```python
from build123d import *

# Parameters (mm, degrees)
BOSS_EXTRUDE4_DEPTH = 50
SKETCH7_R           = 1.75
CUT_EXTRUDE1_DEPTH  = 17.825


with BuildPart() as part:
    # Sketch6 → Boss-Extrude4 (new body)
    with BuildSketch(Plane.XZ):
        with BuildLine():
            Line((-1, 25.784833184), (-1, 12.785954208))
            ThreePointArc((-1, 12.785954208), (-12.825, 0), (-1, -12.785954208))
            Line((-1, -12.785954208), (-1, -25.784833184))
            Line((-1, -25.784833184), (-6, -25.784833184))
            Line((-6, -25.784833184), (-6, -16.784833184))
            ThreePointArc((-6, -16.784833184), (-17.825, 0), (-6, 16.784833184))
            Line((-6, 16.784833184), (-6, 25.784833184))
            Line((-6, 25.784833184), (-1, 25.784833184))
        make_face()
    extrude(amount=BOSS_EXTRUDE4_DEPTH)

    # Sketch7 → Cut-Extrude1 (cut, through all)
    with BuildSketch(Plane(origin=(-1, 0, 0), x_dir=(0, 0, -1), z_dir=(1, 0, 0))):
        with Locations((-19.285393696, -10)):
            Circle(SKETCH7_R)
        with Locations((-19.285393696, -40)):
            Circle(SKETCH7_R)
        with Locations((19.285393696, -40)):
            Circle(SKETCH7_R)
        with Locations((19.285393696, -10)):
            Circle(SKETCH7_R)
    extrude(amount=-CUT_EXTRUDE1_DEPTH, mode=Mode.SUBTRACT)


solid = part.part
```
Geometry: final body of the model. Coordinates: model frame, mm. A direction names the side the tool comes from. Coordinates: 2 decimals unless noted, no trailing zeros. Order: outer loops, then holes, each group sorted by start corner. A loop starts at its lowest first (then second) coordinate and runs counter-clockwise, first axis right, second up. Notation, with made-up numbers: (87, 33.5) - (95, 33.5) arc R12 ccw to (95, 43.5) - close; hole circle Ø11 at (-12.5, 0). An arc over 180 degrees is marked (long way). Write each question's results on one line, items separated by ' | '.
1) Section B-B, the plane x = -9.5. Return loops of the section in (y, z).
Results list:
outline: (-50, -15.08) - (0, -15.08) - (0, -8.62) - (-50, -8.62) - close; (-50, 8.62) - (0, 8.62) - (0, 15.08) - (-50, 15.08) - close
2) Set-up query: faces 4 (the flat face through (-6, -25, 21)), 5 (the cylindrical face through (-3.465, -9.474, -20.955)), 6 (the flat face through (-6, -25, -21)). Return all of +Z, -Z, +X, -X, +Y, -Y with unobstructed straight access to the full face (end or side cutting, diameter ignored); none if empty.
Results list:
face 4: +Z, -X, +Y, -Y | face 5: +X, -X | face 6: -Z, -X, +Y, -Y
3) Line query: line 1 (X direction, y = -28, z = -18); line 2 (Z direction, x = -9, y = -43); line 3 (Z direction, x = -2.75, y = -23). Output: solid intervals per line, ascending. Write a range as from..to.
Results list:
line 1: -6..-1 | line 2: -15.39..-9.14, 9.14..15.39 | line 3: -25.78..-12.53, 12.53..25.78
4) Pull-direction query (Z, two-part tool) for faces 1 (the flat face through (-3, -25, -25.785)), 2 (the cylindrical face through (-3.5, -41.7, 19.7)), 3 (the flat face through (-1, -25, -19)); classes: pulls with the +Z half, pulls with the -Z half, needs draft (parallel to the pull), parting line crosses it, or undercut.
Results list:
face 1: pulls with the -Z half | face 2: undercut | face 3: needs draft
5) Pin query (flat end, axial travel): pin 1 (4 mm diameter, centred on y = -29, z = 13, fed in from -X); pin 2 (4.5 mm diameter, centred on y = -34.5, z = -22, fed in from -X); pin 3 (2 mm diameter, centred on y = -40, z = -19.29, fed in from +X); pin 4 (2 mm diameter, centred on x = -16, y = -32, fed in from -Z). Return the tip coordinate at first contact, or that it passes through.
Results list:
pin 1: x = -14.03 | pin 2: x = -6 | pin 3: through | pin 4: z = -9.63
6) Section A-A, the plane y = -40. Return loops of the section in (x, z) (3 decimals), plus the area to 3 significant figures.
Results list:
outline: (-6, -25.785) - (-1, -25.785) - (-1, -21.035) - (-6, -21.035) - close; (-6, -17.535) - (-1, -17.535) - (-1, -12.786) arc R12.825 cw to (-1, 12.786) - (-1, 17.535) - (-6, 17.535) - (-6, 16.785) arc R17.825 ccw to (-6, -16.785) - close; (-6, 21.035) - (-1, 21.035) - (-1, 25.785) - (-6, 25.785) - close | area: 279 mm^2
7) Section C-C, the plane x = -4.25. Return loops of the section in (y, z), plus the area to 3 significant figures.
Results list:
outline: (-50, -25.78) - (0, -25.78) - (0, -12.1) - (-50, -12.1) - close; (-50, 12.1) - (0, 12.1) - (0, 25.78) - (-50, 25.78) - close; hole circle Ø3.5 at (-40, -19.29); hole circle Ø3.5 at (-40, 19.29); hole circle Ø3.5 at (-10, -19.29); hole circle Ø3.5 at (-10, 19.29) | area: 1,330 mm^2
8) Section D-D, the plane y = -16. Return loops of the section in (x, z) (3 decimals), plus the area to 3 significant figures.
Results list:
outline: (-6, -25.785) - (-1, -25.785) - (-1, -12.786) arc R12.825 cw to (-1, 12.786) - (-1, 25.785) - (-6, 25.785) - (-6, 16.785) arc R17.825 ccw to (-6, -16.785) - close | area: 314 mm^2
